The model under review builds one solid part; all positions refer to its coordinate system, in mm. A direction names the side the tool comes from. Coordinates: 2 decimals unless noted, no trailing zeros. Order: outer loops, then holes, each group sorted by start corner. A loop starts at its lowest first (then second) coordinate and runs counter-clockwise, first axis right, second up. Notation, with made-up numbers: (1, 86.25) -> (28, 86.25) arc R36 cw to (28, 125.25) -> close; hole circle Ø5 at (8, 38). An arc over 180 degrees is marked (long way). Use CSV: the item, a comma, the result in double quotes. Start each with the question number.
```python
from build123d import *

# Parameters (mm, degrees)
EXTRUDE_1_DEPTH              = 5
SKETCH_3_R                   = 2.5
SKETCH_3_R_2                 = 1.75
CUT_EXTRUDE_2_DEPTH          = 78.129760793
EXTRUDE_2_DEPTH              = 32
SKETCH_11_R                  = 1.65
CUT_EXTRUDE_3_DEPTH          = 84.654049513
HOLE_WIZARD_M5_1_D           = 12
HOLE_WIZARD_M5_1_CBORE_D     = 16
HOLE_WIZARD_M5_1_CBORE_DEPTH = 3
FILLET_2_R                   = 3
CUT_EXTRUDE_4_DEPTH          = 82.351090958


with BuildPart() as part:
    # 草图2 → 凸台-拉伸1 (new body)
    with BuildSketch(Plane(origin=(0, 0, 0), x_dir=(1, 0, 0), z_dir=(0, 1, 0))):
        with BuildLine():
            Line((-70, 27), (-70, 10))
            ThreePointArc((-70, 10), (-68.535533906, 6.464466094), (-65, 5))
            Line((-65, 5), (35, 5))
            ThreePointArc((35, 5), (38.535533906, 6.464466094), (40, 10))
            Line((40, 10), (40, 27))
            ThreePointArc((40, 27), (38.535533906, 30.535533906), (35, 32))
            Line((35, 32), (-65, 32))
            ThreePointArc((-65, 32), (-68.535533906, 30.535533906), (-70, 27))
        make_face()
    extrude(amount=EXTRUDE_1_DEPTH)

    # 草图3 → 切除-拉伸2 (cut, through all)
    with BuildSketch(Plane(origin=(0, 5, 0), x_dir=(1, 0, 0), z_dir=(0, 1, 0))):
        with Locations(Location((-34, 26, 0), (0, 0, 270))):
            Circle(SKETCH_3_R)
        with Locations(Location((34, 26, 0), (0, 0, 270))):
            Circle(SKETCH_3_R)
        with Locations(Location((-66, 25, 0), (0, 0, 270))):
            Circle(SKETCH_3_R_2)
    extrude(amount=-CUT_EXTRUDE_2_DEPTH, mode=Mode.SUBTRACT)

    # 草图6 → 凸台-拉伸2 (add)
    with BuildSketch(Plane(origin=(0, 5, 0), x_dir=(1, 0, 0), z_dir=(0, 1, 0))):
        Polygon((-25, 5), (-25, 32), (-19.986167978, 32), (-19.986167978, 10), (19.383137048, 10), (19.383137048, 32), (25, 32), (25, 5), align=None)
    extrude(amount=EXTRUDE_2_DEPTH)

    # 草图11 → 切除-拉伸3 (cut, through all)
    with BuildSketch(Plane.XY.offset(-5)):
        with Locations((-10.82, 29.25)):
            Circle(SKETCH_11_R)
        with Locations((10.82, 29.25)):
            Circle(SKETCH_11_R)
        with Locations((-10.82, 16.75)):
            Circle(SKETCH_11_R)
        with Locations((10.82, 16.75)):
            Circle(SKETCH_11_R)
    extrude(amount=-CUT_EXTRUDE_3_DEPTH, mode=Mode.SUBTRACT)

    # M5 六角头螺钉的柱形沉头孔1 (through all)
    with Locations(Plane(origin=(-0.000886088, 23, -5), x_dir=(1, 0, 0), z_dir=(0, 0, 1))):
        with Locations((0, 0)):
            CounterBoreHole(HOLE_WIZARD_M5_1_D / 2, HOLE_WIZARD_M5_1_CBORE_D / 2, HOLE_WIZARD_M5_1_CBORE_DEPTH)

    # 圆角2
    fillet_2_edges = [part.edges().sort_by_distance(p)[0] for p in [
        (-25, 5, -18.5),
        (19.383137048, 21, -10),
        (-19.986167978, 21, -10),
        (-19.986167978, 5, -21),
        (19.383137048, 5, -21),
        (25, 5, -18.5),
        (-0.301515465, 5, -10),
    ]]
    fillet(fillet_2_edges, radius=FILLET_2_R)

    # 草图18 → 切除-拉伸4 (cut, through all)
    with BuildSketch(Plane.ZY.offset(25)):
        Polygon((-10, 37), (-32, 8), (-32, 37), align=None)
    extrude(amount=-CUT_EXTRUDE_4_DEPTH, mode=Mode.SUBTRACT)


solid = part.part
```
Q1. Clearance check with flat-ended pins moving along their axes: pin 1 Ø9.5 at (x, z) = (-5, -19) entering from +Y; pin 2 Ø12 at (y, z) = (7, -28.5) entering from +X; pin 3 Ø5.5 at (y, z) = (25, -18.5) entering from -X; pin 4 Ø8 at (y, z) = (26, -13) entering from +X. State where each tip first meets the part, or that it passes through.
Q2. Draft analysis for pull direction Y (two halves, no side actions). For faces 1 (the cylindrical face through (1.3, 17.143, -9.014)), 2 (the cylindrical face through (25.9, 5.86, -18.31)), 3 (the flat face through (-19.986, 15, -18)), state which applies: +Y half, -Y half, draft (parallel to the pull), parting line (faces both ways), or undercut.
Q3. Add section A-A, the plane x = 34. State the section outline as (y, z) points, then the cut area to 3 significant figures.
Q4. Add section D-D, the plane y = 25. State the section outline as (x, z) points, then the cut area to 3 significant figures.
Q5. To check wall thickness, follow probe 1 along Y at (x, z) = (-10.5, -8.5); probe 2 along X at (y, z) = (10.5, -23); probe 3 along X at (y, z) = (1.85, -26). State the ranges of each line that lie inside material, in increasing order.
Q6. For faces 4 (the flat face through (34, 5, -19)), 5 (the flat face through (-49, 5, -19)), 6 (the flat face through (-1, 16, -10)), list the 3-axis set-ups (+Z, -Z, +X, -X, +Y, -Y) from which the entire face can be reached by the end or side of a thin tool; tool diameter is ignored.
Q7. Add section C-C, the plane y = 3. State the section outline as (x, z) points.
Q8. Add section B-B, the plane x = -10.82. State the section outline as (y, z) points, then the cut area to 3 significant figures.
Answer block:
1,pin 1,"stops at y = 5"
1,pin 2,"stops at x = 40"
1,pin 3,"stops at x = -25"
1,pin 4,"stops at x = 25"
2,face 1,"undercut"
2,face 2,"+Y half"
2,face 3,"draft"
3,outline,"(0, -32) -> (5, -32) -> (5, -28.5) -> (0, -28.5) -> close; (0, -23.5) -> (5, -23.5) -> (5, -5) -> (0, -5) -> close"
3,area,"110 mm²"
4,outline,"(-25, -19.1) -> (-19.99, -19.1) -> (-19.99, -13) arc R3 cw to (-16.99, -10) -> (-5.66, -10) -> (-5.66, -8) -> (-7.75, -8) -> (-7.75, -5) -> (-25, -5) -> close; (5.66, -10) -> (16.38, -10) arc R3 cw to (19.38, -13) -> (19.38, -19.1) -> (25, -19.1) -> (25, -5) -> (7.75, -5) -> (7.75, -8) -> (5.66, -8) -> close"
4,area,"282 mm²"
5,probe 1,"y = 0 to 15.13, 18.37 to 27.63, 30.87 to 37"
5,probe 2,"x = -25 to -19.99, 19.38 to 25"
5,probe 3,"x = -70 to -67.44, -64.56 to -36.5, -31.5 to 31.5, 36.5 to 40"
6,face 4,"+Z, -Z, +X, +Y"
6,face 5,"+Z, -Z, -X, +Y"
6,face 6,"-Z, +Y"
7,outline,"(-70, -27) arc R5 ccw to (-65, -32) -> (35, -32) arc R5 ccw to (40, -27) -> (40, -10) arc R5 ccw to (35, -5) -> (-65, -5) arc R5 ccw to (-70, -10) -> close; hole circle Ø3.5 at (-66, -25); hole circle Ø5 at (-34, -26); hole circle Ø5 at (34, -26)"
8,outline,"(0, -32) -> (5, -32) -> (5, -13) arc R3 cw to (8, -10) -> (15.1, -10) -> (15.1, -5) -> (0, -5) -> close; (18.4, -10) -> (27.6, -10) -> (27.6, -5) -> (18.4, -5) -> close; (30.9, -10) -> (37, -10) -> (37, -5) -> (30.9, -5) -> close"
8,area,"264 mm²"
